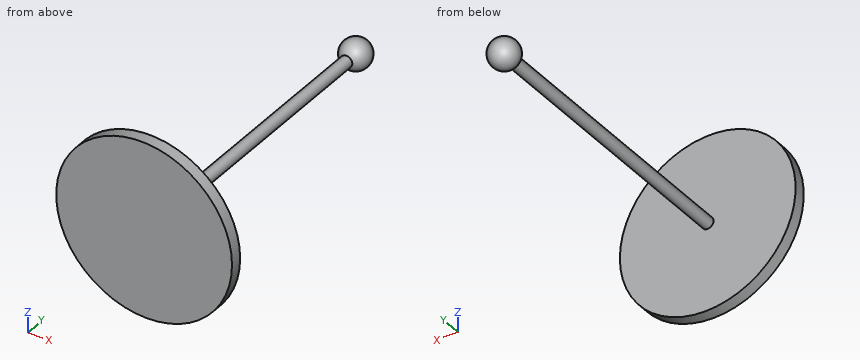
from build123d import *

# Parameters (mm, degrees)
ESBO_O1_R                = 75
RESSALTO_EXTRUS_O1_DEPTH = 10
ESBO_O2_R                = 5
RESSALTO_EXTRUS_O2_DEPTH = 250


with BuildPart() as part:
    # Esboço1 → Ressalto-extrusão1 (new body)
    with BuildSketch(Plane(origin=(0, 0, 0), x_dir=(1, 0, 0), z_dir=(0, 1, 0))):
        Circle(ESBO_O1_R)
    extrude(amount=RESSALTO_EXTRUS_O1_DEPTH)

    # Esboço2 → Ressalto-extrusão2 (add)
    with BuildSketch(Plane(origin=(0, 10, 0), x_dir=(1, 0, 0), z_dir=(0, 1, 0))):
        Circle(ESBO_O2_R)
    extrude(amount=RESSALTO_EXTRUS_O2_DEPTH)

    # Esboço4 → Revolução1 (revolve)
    with BuildSketch(Plane(origin=(0, 0, 0), x_dir=(0, 0, -1), z_dir=(1, 0, 0))):
        with BuildLine():
            Line((0, 272.5), (0, 247.5))
            ThreePointArc((0, 247.5), (12.5, 260), (0, 272.5))
        make_face()
    revolve(axis=Axis((0, 272.5, 0), (0, -1, 0)))


solid = part.part
The model under review builds one solid part; all positions refer to its coordinate system, in mm. Round coordinates to 2 decimals unless told otherwise and drop trailing zeros. Write each loop counter-clockwise with the first axis right and the second up, starting at its lowest first coordinate (ties: lowest second). Pieces come first, ordered by that corner, then holes. Notation, with made-up numbers: M 4.25,65 L 52.25,65 A15 ccw 52.25,94 Z; hole C 69,5.5 d7. An arc over 180 degrees is marked long. Use a Markdown table: item, result. Add a question column.
Q1. Insertion check: pin 1 (12 mm diameter, centred on y = 95, z = -8.5, fed in from +X); pin 2 (10 mm diameter, centred on y = 171, z = -9, fed in from -X). Each pin has a flat end and moves straight along its axis. Give the tip position at first contact, or say it passes through.
Q2. We need section C-C, the plane y = 145.5. State the section outline as (x, z) points, plus the area to 3 significant figures.
Q3. We need section B-B, the plane x = 0. State the section outline as (y, z) points.
Q4. We need section D-D, the plane z = -23.5. State the section outline as (x, y) points.
Q5. To check wall thickness, follow line 1 (Y direction, x = -9, z = -22.5); line 2 (X direction, y = 91.5, z = -3). State the ranges of each line that lie inside material, in increasing order.
Q6. We need section A-A, the plane z = 0. State the section outline as (x, y) points, plus the area to 3 significant figures.
Findings below:
| question | item | result |
|---|---|---|
| 1 | pin 1 | stops at x = 4.33 |
| 1 | pin 2 | stops at x = -3 |
| 2 | outline | C 0,0 d10 |
| 2 | area | 78.5 mm² |
| 3 | outline | M 0,-75 L 10,-75 L 10,-5 L 248.54,-5 A12.5 ccw long 248.54,5 L 10,5 L 10,75 L 0,75 Z |
| 4 | outline | M -71.22,0 L 71.22,0 L 71.22,10 L -71.22,10 Z |
| 5 | line 1 | y = 0 to 10 |
| 5 | line 2 | x = -4 to 4 |
| 6 | outline | M -75,0 L 75,0 L 75,10 L 5,10 L 5,248.54 A12.5 ccw long -5,248.54 L -5,10 L -75,10 Z |
| 6 | area | 4,370 mm² |
